The model under review builds one solid part; all positions refer to its coordinate system, in mm. Coordinates: 2 decimals unless noted, no trailing zeros. Order: outer loops, then holes, each group sorted by start corner. A loop starts at its lowest first (then second) coordinate and runs counter-clockwise, first axis right, second up. Notation, with made-up numbers: (76, -17.5) - (82, -17.5) arc R27 ccw to (82, 16.5) - close; hole circle Ø7 at (53, 3.25). An arc over 180 degrees is marked (long way). Answer in a Markdown table with one row per item.
```python
from build123d import *

# Parameters (mm, degrees)
SKETCH1_W           = 78
SKETCH1_H           = 118
BOSS_EXTRUDE1_DEPTH = 1
SKETCH2_R           = 2
SKETCH2_R_2         = 1.5
CUT_EXTRUDE1_DEPTH  = 142.453172464


with BuildPart() as part:
    # Sketch1 → Boss-Extrude1 (new body)
    with BuildSketch(Plane.XY):
        with Locations((39, 59)):
            Rectangle(SKETCH1_W, SKETCH1_H)
    extrude(amount=BOSS_EXTRUDE1_DEPTH)

    # Sketch2 → Cut-Extrude1 (cut, through all)
    with BuildSketch(Plane(origin=(0, 0, 0), x_dir=(-1, 0, 0), z_dir=(0, 0, -1))):
        with Locations((-8.980393049, 39.016810723)):
            Circle(SKETCH2_R)
        with Locations((-68.980393049, 39.016810723)):
            Circle(SKETCH2_R)
        with Locations((-68.980393049, 109.016810723)):
            Circle(SKETCH2_R)
        with Locations((-8.980393049, 109.016810723)):
            Circle(SKETCH2_R)
        with Locations((-66, 12)):
            Circle(SKETCH2_R_2)
        with Locations((-60, 12)):
            Circle(SKETCH2_R_2)
        with Locations((-54, 12)):
            Circle(SKETCH2_R_2)
        with Locations((-48, 12)):
            Circle(SKETCH2_R_2)
        with Locations((-42, 12)):
            Circle(SKETCH2_R_2)
        with Locations((-36, 12)):
            Circle(SKETCH2_R_2)
        with Locations((-30, 12)):
            Circle(SKETCH2_R_2)
        with Locations((-24, 12)):
            Circle(SKETCH2_R_2)
        with Locations((-18, 12)):
            Circle(SKETCH2_R_2)
        with Locations((-12, 12)):
            Circle(SKETCH2_R_2)
        with Locations((-60, 6)):
            Circle(SKETCH2_R_2)
        with Locations((-54, 6)):
            Circle(SKETCH2_R_2)
        with Locations((-48, 6)):
            Circle(SKETCH2_R_2)
        with Locations((-42, 6)):
            Circle(SKETCH2_R_2)
        with Locations((-36, 6)):
            Circle(SKETCH2_R_2)
        with Locations((-30, 6)):
            Circle(SKETCH2_R_2)
        with Locations((-24, 6)):
            Circle(SKETCH2_R_2)
        with Locations((-18, 6)):
            Circle(SKETCH2_R_2)
        with Locations((-12, 6)):
            Circle(SKETCH2_R_2)
        with Locations((-66, 6)):
            Circle(SKETCH2_R_2)
    extrude(amount=-CUT_EXTRUDE1_DEPTH, mode=Mode.SUBTRACT)


solid = part.part
```
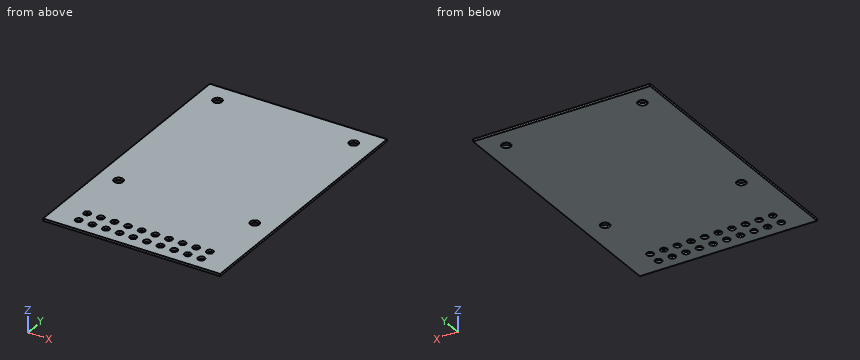
Item 1: To check wall thickness, follow line 1 (Y direction, x = 54, z = 0.55); line 2 (Y direction, x = 55, z = 0.85). State the ranges of each line that lie inside material, in increasing order. Write a range as from..to.
Check values:
| item | result |
|---|---|
| line 1 | 0..4.5, 7.5..10.5, 13.5..118 |
| line 2 | 0..4.88, 7.12..10.88, 13.12..118 |
Item 2: We need section B-B, the plane z = 0.7. State how many separate pieces and enclosed holes the cut face has, then the cut area to 3 significant figures.
Check values:
| item | result |
|---|---|
| separate pieces | 1 |
| enclosed holes | 24 |
| area | 9,010 mm^2 |
Item 3: We need section A-A, the plane x = 30. Write out the cut boundary in (y, z).
Check values:
| item | result |
|---|---|
| outline | (0, 0) - (4.5, 0) - (4.5, 1) - (0, 1) - close; (7.5, 0) - (10.5, 0) - (10.5, 1) - (7.5, 1) - close; (13.5, 0) - (118, 0) - (118, 1) - (13.5, 1) - close |
Item 4: Clearance check with a flat-ended pin moving along its axis: pin 1 Ø2.5 at (x, y) = (18, 12) entering from +Z. State where the tip first meets the part, or that it passes through.
Check values:
| item | result |
|---|---|
| pin 1 | through |
